Design review of the part built by this model. Coordinates are the model's own, in mm. Face numbers are marked on the shaded views. A direction names the side the tool comes from. Coordinates: 2 decimals unless noted, no trailing zeros. Order: outer loops, then holes, each group sorted by start corner. A loop starts at its lowest first (then second) coordinate and runs counter-clockwise, first axis right, second up.
from build123d import *
from build123d.topology import SkipClean

# Parameters (mm, degrees)
SKETCH1_W                = 39
SKETCH1_H                = 7.38
BOSS_EXTRUDE1_DEPTH      = 7.76
SKETCH2_R                = 2.4
CUT_EXTRUDE1_DEPTH       = 7.76
CUT_EXTRUDE2_OUTLINE_R   = 3.1
CUT_EXTRUDE2_OUTLINE_R_2 = 2.4
CUT_EXTRUDE2_DEPTH       = 0.8
CUT_EXTRUDE3_START       = 6.96
CUT_EXTRUDE3_OUTLINE_R   = 3.1
CUT_EXTRUDE3_OUTLINE_R_2 = 2.4
CUT_EXTRUDE3_DEPTH       = 0.8
LPATTERN3_COUNT          = 3
LPATTERN3_PITCH          = 7.79
LPATTERN6_COUNT          = 3
LPATTERN6_PITCH          = 7.79
FILLET1_R                = 3.69
FILLET2_R                = 3.69
FILLET3_R                = 3.69
FILLET4_R                = 3.69
SCALE1_SCALE             = 1.03
SKETCH5_R                = 3.193
BOSS_EXTRUDE2_DEPTH      = 7.99
SKETCH7_W                = 16
SKETCH7_H                = 7.6014
BOSS_EXTRUDE4_DEPTH      = 7.99
SKETCH4_R                = 1.59
BOSS_EXTRUDE5_DEPTH      = 6
FILLET5_R                = 4
FILLET6_R                = 4
FILLET7_R                = 4
FILLET8_R                = 4


with BuildPart() as part:
    # Sketch1 → Boss-Extrude1 (new body)
    with BuildSketch(Plane.XY):
        with Locations((19.5, 3.69)):
            Rectangle(SKETCH1_W, SKETCH1_H)
    extrude(amount=BOSS_EXTRUDE1_DEPTH)

    # Sketch2 → Cut-Extrude1 (cut)
    with BuildSketch(Plane.XY.offset(7.76)):
        with Locations((19.5, 3.69)):
            Circle(SKETCH2_R)
    cut_extrude1 = extrude(amount=-CUT_EXTRUDE1_DEPTH, mode=Mode.SUBTRACT)

    # Cut-Extrude2: read off the stored shape, not the designer's step
    # Cut-Extrude2 outline → Cut-Extrude2 (cut)
    with BuildSketch(Plane.XY):
        with Locations((19.5, 3.69)):
            Circle(CUT_EXTRUDE2_OUTLINE_R)
        with Locations((19.5, 3.69)):
            Circle(CUT_EXTRUDE2_OUTLINE_R_2, mode=Mode.SUBTRACT)
    cut_extrude2 = extrude(amount=CUT_EXTRUDE2_DEPTH, mode=Mode.SUBTRACT)

    # Cut-Extrude3: read off the stored shape, not the designer's step
    # Cut-Extrude3 outline → Cut-Extrude3 (cut)
    with BuildSketch(Plane.XY.offset(CUT_EXTRUDE3_START)):
        with Locations((19.5, 3.69)):
            Circle(CUT_EXTRUDE3_OUTLINE_R)
        with Locations((19.5, 3.69)):
            Circle(CUT_EXTRUDE3_OUTLINE_R_2, mode=Mode.SUBTRACT)
    cut_extrude3 = extrude(amount=CUT_EXTRUDE3_DEPTH, mode=Mode.SUBTRACT)

    # LPattern3: Cut-Extrude1, Cut-Extrude2, Cut-Extrude3 ×3
    with Locations(*[(-i * LPATTERN3_PITCH, 0, 0) for i in range(1, LPATTERN3_COUNT)]):
        add(cut_extrude1, mode=Mode.SUBTRACT)
        add(cut_extrude2, mode=Mode.SUBTRACT)
        add(cut_extrude3, mode=Mode.SUBTRACT)

    # LPattern6: Cut-Extrude1, Cut-Extrude2, Cut-Extrude3 ×3
    with Locations(*[(i * LPATTERN6_PITCH, 0, 0) for i in range(1, LPATTERN6_COUNT)]):
        add(cut_extrude1, mode=Mode.SUBTRACT)
        add(cut_extrude2, mode=Mode.SUBTRACT)
        add(cut_extrude3, mode=Mode.SUBTRACT)

    # Fillet1
    fillet1_edges = [part.edges().sort_by_distance(p)[0] for p in [
        (0, 7.38, 3.88),
    ]]
    fillet(fillet1_edges, radius=FILLET1_R)

    # Fillet2
    fillet2_edges = [part.edges().sort_by_distance(p)[0] for p in [
        (0, 0, 3.88),
    ]]
    fillet(fillet2_edges, radius=FILLET2_R - 0.0001)  # a hair under: the kernel refuses the full size

    # Fillet3
    fillet3_edges = [part.edges().sort_by_distance(p)[0] for p in [
        (39, 7.38, 3.88),
    ]]
    fillet(fillet3_edges, radius=FILLET3_R)

    # Fillet4
    fillet4_edges = [part.edges().sort_by_distance(p)[0] for p in [
        (39, 0, 3.88),
    ]]
    fillet(fillet4_edges, radius=FILLET4_R - 0.0001)  # a hair under: the kernel refuses the full size


with BuildPart() as part_1:
    # Scale1: scaled about (19.5, 3.689995512, 3.88)
    add(part.part.scale(SCALE1_SCALE).moved(Location((-0.585, -0.110699865, -0.1164))))

    # Sketch5 → Boss-Extrude2 (add)
    with BuildSketch(Plane(origin=(0, 0, -0.1164), x_dir=(-1, 0, 0), z_dir=(0, 0, -1))):
        with Locations((-35.5474, 3.69)):
            Circle(SKETCH5_R)
        with Locations((-3.4526, 3.69)):
            Circle(SKETCH5_R)
    extrude(amount=-BOSS_EXTRUDE2_DEPTH)

    # Sketch7 → Boss-Extrude4 (add)
    with SkipClean():  # the faces are left unmerged after this step: merging them gives an invalid solid
        with BuildSketch(Plane(origin=(0, 0, -0.1164), x_dir=(-1, 0, 0), z_dir=(0, 0, -1))):
            with Locations((-43.7843, 3.69)):
                Rectangle(SKETCH7_W, SKETCH7_H)
            with Locations((4.7843, 3.69)):
                Rectangle(SKETCH7_W, SKETCH7_H)
        extrude(amount=-BOSS_EXTRUDE4_DEPTH)

    # Sketch4 → Boss-Extrude5 (add)
    with SkipClean():  # the faces are left unmerged after this step: merging them gives an invalid solid
        with BuildSketch(Plane(origin=(0, 0, -0.1164), x_dir=(-1, 0, 0), z_dir=(0, 0, -1))):
            with Locations((-47.1, 3.69)):
                Circle(SKETCH4_R)
            with Locations((8.1, 3.69)):
                Circle(SKETCH4_R)
        extrude(amount=BOSS_EXTRUDE5_DEPTH)

    # Fillet5
    fillet5_edges = [part_1.edges().sort_by_distance(p)[0] for p in [
        (51.7843, -0.1107, 3.8786),
    ]]
    fillet(fillet5_edges, radius=FILLET5_R)

    # Fillet6
    # the kernel refuses this fillet: 4 mm, written as the material it takes off along each edge
    with BuildSketch(Plane(origin=(51.7843, 7.4907, -10.066625513), x_dir=(0, -1, 0), z_dir=(0, 0, 1))) as fillet6_piece_1:
        with BuildLine():
            CenterArc((4, -3.980090205), FILLET6_R, 95.719016284, 84.280983716)
            Line((0, -3.980090205), (-0.08, -3.980090205))
            Line((-0.08, -3.980090205), (-0.08, 0))
            Line((-0.08, 0), (0, 0.08))
            ThreePointArc((0, 0.08), (1.8007, 0.08), (3.593428, 0.079601804))
            Line((3.593428, 0.079601804), (3.6014, 0))
        make_face()
    extrude(amount=27.890451025, mode=Mode.SUBTRACT)

    # Fillet7
    fillet7_edges = [part_1.edges().sort_by_distance(p)[0] for p in [
        (-12.7843, 7.4907, 3.8786),
    ]]
    fillet(fillet7_edges, radius=FILLET7_R)

    # Fillet8
    # the kernel refuses this fillet: 4 mm, written as the material it takes off along each edge
    with BuildSketch(Plane(origin=(-12.7843, -0.1107, -10.066625513), x_dir=(0, 1, 0), z_dir=(0, 0, 1))) as fillet8_piece_1:
        with BuildLine():
            CenterArc((4, -3.980090205), FILLET8_R, 95.719016284, 84.280983716)
            Line((0, -3.980090205), (-0.08, -3.980090205))
            Line((-0.08, -3.980090205), (-0.08, 0))
            Line((-0.08, 0), (0, 0.08))
            ThreePointArc((0, 0.08), (1.8007, 0.08), (3.593428, 0.079601804))
            Line((3.593428, 0.079601804), (3.6014, 0))
        make_face()
    extrude(amount=27.890451025, mode=Mode.SUBTRACT)


solid = part_1.part
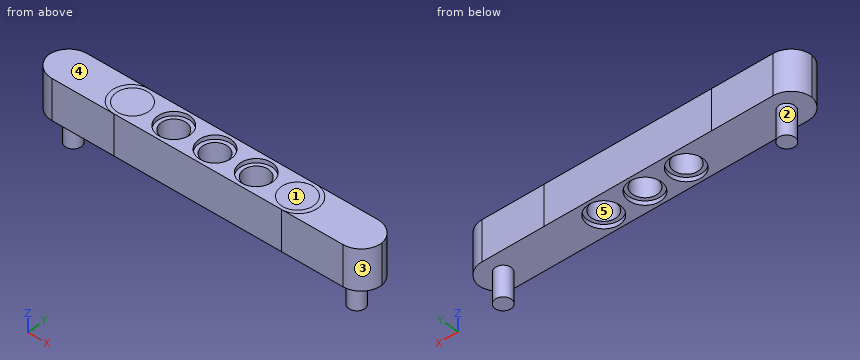
1. Add section B-B (z = 6). Give the boundary of the cut face in (x, y).
2. Add section D-D (x = 29). Give the boundary of the cut face in (y, z), and give its area (3 significant figures).
3. Insertion check: pin 1 (3 mm diameter, centred on x = 12.5, y = 4.5, fed in from +Z); pin 2 (5 mm diameter, centred on x = -6, z = -4, fed in from -Y); pin 3 (4 mm diameter, centred on x = 3.45, y = 3.69, fed in from +Z). Each pin has a flat end and moves straight along its axis. Give the tip position at first contact, or say it passes through.
4. To check wall thickness, follow line 1 (X direction, y = 2.25, z = 3.25); line 2 (Y direction, x = 19.5, z = 4.75); line 3 (X direction, y = 3.25, z = 4.75). State the ranges of each line that lie inside material, in increasing order.
5. For the marked faces 1 and 2, list the 3-axis set-ups (+Z, -Z, +X, -X, +Y, -Y) from which the entire face can be reached by the end or side of a thin tool; tool diameter is ignored.
6. Mouldability with a two-part tool opening along Y and no side actions: class the marked faces 3, 4 and 5 as pulls with the +Y half, pulls with the -Y half, needs draft (parallel to the pull), parting line crosses it, or undercut.
7. Add section C-C (z = -4.75). Give the boundary of the cut face in (x, y).
8. Add section A-A (x = 19.5). Give the boundary of the cut face in (y, z), and give its area (3 significant figures).
Solution:
1. outline: (-12.78, 3.49) arc R4 ccw to (-8.8, -0.11) - (47.78, -0.11) arc R4 ccw to (51.78, 3.89) arc R4 ccw to (47.8, 7.49) - (-8.78, 7.49) arc R4 ccw to start; hole circle Ø4.94 at (11.48, 3.69); hole circle Ø4.94 at (19.5, 3.69); hole circle Ø4.94 at (27.52, 3.69)
2. outline: (-0.11, -0.12) - (0.86, -0.12) - (0.86, 0.71) - (1.71, 0.71) - (1.71, 7.05) - (0.86, 7.05) - (0.86, 7.88) - (-0.11, 7.88) - close; (5.67, 0.71) - (6.52, 0.71) - (6.52, -0.12) - (7.49, -0.12) - (7.49, 7.88) - (6.52, 7.88) - (6.52, 7.05) - (5.67, 7.05) - close
2. area: 26.3 mm2
3. pin 1: stops at z = 7.05
3. pin 2: stops at y = 2.1
3. pin 3: stops at z = 7.87
4. line 1: x = -12.45 to 9.47, 13.49 to 17.49, 21.51 to 25.51, 29.53 to 51.43
4. line 2: y = -0.11 to 1.22, 6.16 to 7.49
4. line 3: x = -12.75 to 9.04, 13.91 to 17.07, 21.93 to 25.09, 29.96 to 51.73
5. face 1: +Z, +X, -X, +Y, -Y
5. face 2: -Z
6. face 3: pulls with the -Y half
6. face 4: needs draft
6. face 5: undercut
7. outline: circle Ø3.18 at (-8.1, 3.69); circle Ø3.18 at (47.1, 3.69)
8. outline: (-0.11, -0.12) - (0.5, -0.12) - (0.5, 0.71) - (1.22, 0.71) - (1.22, 7.05) - (0.5, 7.05) - (0.5, 7.88) - (-0.11, 7.88) - close; (6.16, 0.71) - (6.88, 0.71) - (6.88, -0.12) - (7.49, -0.12) - (7.49, 7.88) - (6.88, 7.88) - (6.88, 7.05) - (6.16, 7.05) - close
8. area: 18.9 mm2
